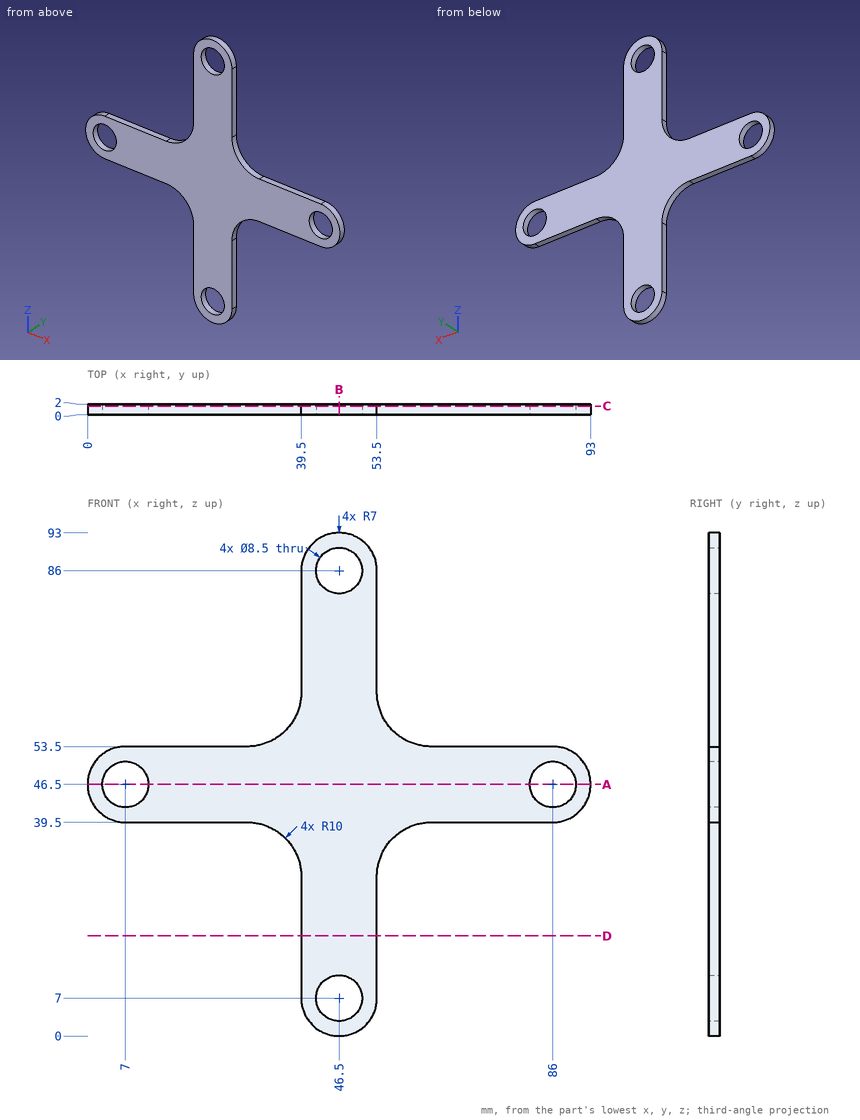
The drawing under review shows one solid part. Ordinate dimensions are in mm from its lowest x, y, z. Round coordinates to 2 decimals unless told otherwise and drop trailing zeros. Loops run counter-clockwise (first coordinate to the right, second up) from the corner with the lowest first, then second, coordinate; pieces in that order, holes last. Notation, with made-up numbers: (70, 59.5) -> (103, 59.5) arc R10 ccw to (103, 66.5) -> close; hole circle Ø3 at (33.25, 8). An arc over 180 degrees is marked (long way). Answer in a Markdown table with one row per item.
1) Consider section B-B, the plane x = 46.5. Write out the cut boundary in (y, z).
Taken from the geometry:
| item | result |
|---|---|
| outline | (0, 0) -> (2, 0) -> (2, 2.75) -> (0, 2.75) -> close; (0, 11.25) -> (2, 11.25) -> (2, 81.75) -> (0, 81.75) -> close; (0, 90.25) -> (2, 90.25) -> (2, 93) -> (0, 93) -> close |
2) Wall thickness on line 1 along X through (y, z) = (0.55, 46.5); line 2 along Z through (x, y) = (23, 0.7); line 3 along X through (y, z) = (0.75, 49): over which ranges is each line inside the solid? List them lowest first.
Taken from the geometry:
| item | result |
|---|---|
| line 1 | x = 0 to 2.75, 11.25 to 81.75, 90.25 to 93 |
| line 2 | z = 39.5 to 53.5 |
| line 3 | x = 0.46 to 3.56, 10.44 to 82.56, 89.44 to 92.54 |
3) Consider section D-D, the plane z = 18.5. Write out the cut boundary in (x, y), plus the area to 3 significant figures.
Taken from the geometry:
| item | result |
|---|---|
| outline | (39.5, 0) -> (53.5, 0) -> (53.5, 2) -> (39.5, 2) -> close |
| area | 28.0 mm² |
4) For pin 1 Ø1 at (y, z) = (0.5, 22.5) entering from +X; pin 2 Ø0.6 at (x, y) = (70, 1) entering from -Z; pin 3 Ø0.6 at (x, y) = (22, 1.5) entering from +Z, all flat-tipped, find the tip position at first contact; note any pin that passes through.
Taken from the geometry:
| item | result |
|---|---|
| pin 1 | stops at x = 53.5 |
| pin 2 | stops at z = 39.5 |
| pin 3 | stops at z = 53.5 |
5) Consider section C-C, the plane y = 1.6. Write out the cut boundary in (x, z), plus the area to 3 significant figures.
Taken from the geometry:
| item | result |
|---|---|
| outline | (7, 39.5) -> (29.5, 39.5) arc R10 cw to (39.5, 29.5) -> (39.5, 7) arc R7 ccw to (53.5, 7) -> (53.5, 29.5) arc R10 cw to (63.5, 39.5) -> (86, 39.5) arc R7 ccw to (86, 53.5) -> (63.5, 53.5) arc R10 cw to (53.5, 63.5) -> (53.5, 86) arc R7 ccw to (39.5, 86) -> (39.5, 63.5) arc R10 cw to (29.5, 53.5) -> (7, 53.5) arc R7 ccw to start; hole circle Ø8.5 at (7, 46.5); hole circle Ø8.5 at (46.5, 7); hole circle Ø8.5 at (46.5, 86); hole circle Ø8.5 at (86, 46.5) |
| area | 2,180 mm² |
6) Consider section A-A, the plane z = 46.5. Write out the cut boundary in (x, y).
Taken from the geometry:
| item | result |
|---|---|
| outline | (0, 0) -> (2.75, 0) -> (2.75, 2) -> (0, 2) -> close; (11.25, 0) -> (81.75, 0) -> (81.75, 2) -> (11.25, 2) -> close; (90.25, 0) -> (93, 0) -> (93, 2) -> (90.25, 2) -> close |
